from build123d import *

# Parameters (mm, degrees)
F0_R     = 2.5
F0_R_2   = 10
F0_R_3   = 6
F1_DEPTH = 25


with BuildPart() as f1:
    # F0 (on Front) → F1 (new body)
    with BuildSketch(Plane.XZ):
        Polygon((-20.799367, 29.298078), (-60.799367, 29.298078), (-60.799367, -10.701922), (19.200633, -10.701922), (19.200633, 9.298078), (-20.799367, 9.298078), align=None)
        with Locations((-55.299367, -5.201922)):
            Circle(F0_R, mode=Mode.SUBTRACT)
        with Locations((-26.299367, -5.201922)):
            Circle(F0_R, mode=Mode.SUBTRACT)
        with Locations((-40.799367, 8.787482)):
            Circle(F0_R_2, mode=Mode.SUBTRACT)
        with Locations((6.200633, -0.701922)):
            Circle(F0_R_3, mode=Mode.SUBTRACT)
        with Locations((-55.299367, 23.798078)):
            Circle(F0_R, mode=Mode.SUBTRACT)
        with Locations((-26.299367, 23.798078)):
            Circle(F0_R, mode=Mode.SUBTRACT)
    extrude(amount=F1_DEPTH)


solid = f1.part
The listing builds one solid part. Answer for the finished solid, in the listing's coordinates (mm). A direction names the side the tool comes from. Coordinates: 2 decimals unless noted, no trailing zeros. Loops run counter-clockwise (first coordinate to the right, second up) from the corner with the lowest first, then second, coordinate; pieces in that order, holes last. Notation, with made-up numbers: M 19.25,51 L 35.25,51 A9 ccw 35.25,64 Z; hole C 16,14.25 d2. An arc over 180 degrees is marked long. Answer in a Markdown table with one row per item.
1) Which of the six approach directions +Z, -Z, +X, -X, +Y, -Y give full straight-line access (tool end or side, diameter ignored) to faces 4 (the flat face through (-1, -12, 9.298)), 5 (the cylindrical face through (4.9, -12.32, -6.56))?
Answers below:
| item | result |
|---|---|
| face 4 | +Z, +X, +Y, -Y |
| face 5 | +Y, -Y |
2) Find the intervals of material crossed by probe 1 along Z at (x, y) = (-26, -17.25); probe 2 along Z at (x, y) = (-40.5, -12.25); probe 3 along X at (y, z) = (-13, -6), in increasing order.
Answers below:
| item | result |
|---|---|
| probe 1 | -10.7 to -7.68, -2.72 to 21.32, 26.28 to 29.3 |
| probe 2 | -10.7 to -1.21, 18.78 to 29.3 |
| probe 3 | -60.8 to -57.67, -52.93 to -28.67, -23.93 to 3.38, 9.02 to 19.2 |
3) Determine the mould class of faces 1 (the cylindrical face through (-50.79, -12.32, 9.23)), 2 (the flat face through (-60.799, -12, 10)), 3 (the flat face through (-41, -12, 29.298)) for opening direction Z: released by +Z, released by -Z, zero draft, split by the parting line, or undercut.
Answers below:
| item | result |
|---|---|
| face 1 | undercut |
| face 2 | zero draft |
| face 3 | released by +Z |
4) Find section A-A (z = 14). Determine the outline of the cut face in (x, y), then the cut area to 3 significant figures.
Answers below:
| item | result |
|---|---|
| outline | M -60.8,-25 L -49.33,-25 L -49.33,0 L -60.8,0 Z; M -32.27,-25 L -20.8,-25 L -20.8,0 L -32.27,0 Z |
| area | 573 mm^2 |
5) Find section D-D (y = -16.25). Determine the outline of the cut face in (x, z).
Answers below:
| item | result |
|---|---|
| outline | M -60.8,-10.7 L 19.2,-10.7 L 19.2,9.3 L -20.8,9.3 L -20.8,29.3 L -60.8,29.3 Z; hole C -55.3,-5.2 d5; hole C -55.3,23.8 d5; hole C -40.8,8.79 d20; hole C -26.3,-5.2 d5; hole C -26.3,23.8 d5; hole C 6.2,-0.7 d12 |
6) Find section C-C (z = 1). Determine the outline of the cut face in (x, y).
Answers below:
| item | result |
|---|---|
| outline | M -60.8,-25 L -47.07,-25 L -47.07,0 L -60.8,0 Z; M -34.53,-25 L 0.45,-25 L 0.45,0 L -34.53,0 Z; M 11.95,-25 L 19.2,-25 L 19.2,0 L 11.95,0 Z |
7) Given pin 1 (6.5 mm diameter, centred on x = -55.3, z = 23.8, fed in from -Y); pin 2 (3 mm diameter, centred on x = -26.3, z = 23.8, fed in from -Y); pin 3 (10 mm diameter, centred on x = 2, y = -11.5, fed in from +Z); pin 4 (10 mm diameter, centred on y = -15, z = 21, fed in from +X), each flat-ended and moving along its own axis, determine where each tip first touches the part or whether it passes through.
Answers below:
| item | result |
|---|---|
| pin 1 | y = -25 |
| pin 2 | through |
| pin 3 | z = 9.3 |
| pin 4 | x = -20.8 |
8) Find section B-B (x = 4). Determine the outline of the cut face in (y, z), then the cut area to 3 significant figures.
Answers below:
| item | result |
|---|---|
| outline | M -25,-10.7 L 0,-10.7 L 0,-6.28 L -25,-6.28 Z; M -25,4.88 L 0,4.88 L 0,9.3 L -25,9.3 Z |
| area | 221 mm^2 |
